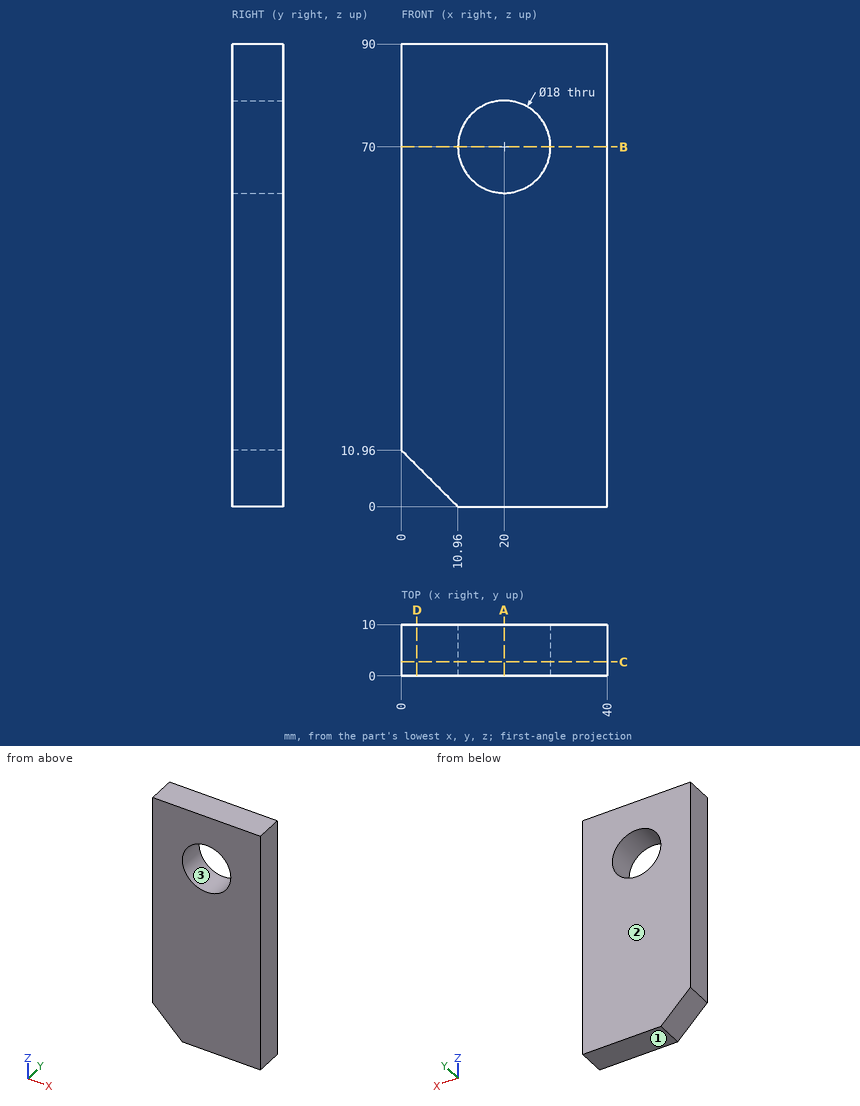
Study the drawing (mm; zero at the part's minimum x, y, z) and answer. Round coordinates to 2 decimals unless told otherwise and drop trailing zeros. Order: outer loops, then holes, each group sorted by start corner. A loop starts at its lowest first (then second) coordinate and runs counter-clockwise, first axis right, second up. Notation, with made-up numbers: (25, 13.5) -> (49, 13.5) arc R25 ccw to (49, 25.5) -> close; hole circle Ø1 at (-26, 85). An arc over 180 degrees is marked (long way). Answer as CSV lines item,"result". Start each with the question number.
(1) The part is cut by section A-A (x = 20). Determine the outline of the cut face in (y, z), then the cut area to 3 significant figures.
(2) For a pull along Z with two mould halves and no side action, classify the marked faces 1, 2 and 3 as +Z half, -Z half, draft (parallel to the pull), parting line (faces both ways), or undercut.
(3) The part is cut by section D-D (x = 3). Determine the outline of the cut face in (y, z).
(4) The part is cut by section B-B (z = 70). Determine the outline of the cut face in (x, y).
(5) The part is cut by section C-C (y = 2.75). Determine the outline of the cut face in (x, z).
(6) A flat-ended cylindrical pin translates along its axis: pin 1 Ø3 at (x, y) = (8, 2.5) entering from -Z. Find the tip coordinate at first contact, or state that the pin passes through.
(7) Find the intervals of material crossed by probe 1 along Z at (x, y) = (20, 4); probe 2 along X at (y, z) = (4.25, 66); probe 3 along Z at (x, y) = (2.5, 9.25), in increasing order. Write a range as from..to.
Evaluation:
1,outline,"(0, 0) -> (10, 0) -> (10, 61) -> (0, 61) -> close; (0, 79) -> (10, 79) -> (10, 90) -> (0, 90) -> close"
1,area,"720 mm²"
2,face 1,"-Z half"
2,face 2,"draft"
2,face 3,"undercut"
3,outline,"(0, 7.96) -> (10, 7.96) -> (10, 90) -> (0, 90) -> close"
4,outline,"(0, 0) -> (11, 0) -> (11, 10) -> (0, 10) -> close; (29, 0) -> (40, 0) -> (40, 10) -> (29, 10) -> close"
5,outline,"(0, 10.96) -> (10.96, 0) -> (40, 0) -> (40, 90) -> (0, 90) -> close; hole circle Ø18 at (20, 70)"
6,pin 1,"z = 1.46"
7,probe 1,"0..61, 79..90"
7,probe 2,"0..11.94, 28.06..40"
7,probe 3,"8.46..90"
